Geometry check sheet. Reference: the model listing, model coordinates, mm. A direction names the side the tool comes from. Round coordinates to 2 decimals unless told otherwise and drop trailing zeros. Write each loop counter-clockwise with the first axis right and the second up, starting at its lowest first coordinate (ties: lowest second). Pieces come first, ordered by that corner, then holes.
from build123d import *

# Parameters (mm, degrees)
BOSS_EXTRUDE1_DEPTH = 18


with BuildPart() as part:
    # Sketch1 → Boss-Extrude1 (new body)
    with BuildSketch(Plane(origin=(0, 0, 0), x_dir=(1, 0, 0), z_dir=(0, 1, 0))):
        with BuildLine():
            Line((66.981499187, 102), (316.981499187, 102))
            Line((316.981499187, 102), (316.981499187, -38))
            Line((316.981499187, -38), (-83.018500813, -38))
            Line((-83.018500813, -38), (-83.018500813, 0))
            Line((-83.018500813, 0), (41.981499187, 0))
            ThreePointArc((41.981499187, 0), (59.659168717, 7.32233047), (66.981499187, 25))
            Line((66.981499187, 25), (66.981499187, 102))
        make_face()
    extrude(amount=BOSS_EXTRUDE1_DEPTH)


solid = part.part
1. Depth check by flat-ended pin: pin 1 Ø9 at (y, z) = (9.5, -77) entering from -X; pin 2 Ø10 at (x, z) = (160, 10) entering from -Y; pin 3 Ø8 at (x, z) = (-18.5, -7.5) entering from -Y. Enter the tip coordinate at first touch or a pass-through.
2. Section check B-B (x = 33). Record the cut outline in (y, z), plus the area to 3 significant figures.
3. Section check A-A (y = 11). Record the cut outline in (x, z), plus the area to 3 significant figures.
4. Section check C-C (z = -55.5). Record the cut outline in (x, y).
5. Access from +Z, -Z, +X, -X, +Y, -Y to the whole of each face (thin tool, end or side, straight path). Record for faces 1 (the face through (316.981, 9, -33)), 2 (the face through (66.981, 9, -63)).
6. Scan lines: line 1 along Z through (x, y) = (-47, 8); line 2 along X through (y, z) = (16.25, -27); line 3 along X through (y, z) = (7.25, -5). Record each from-to range of solid material in increasing order.
Results below:
1. pin 1: stops at x = 66.98
1. pin 2: stops at y = 0
1. pin 3: passes through
2. outline: (0, 0) - (18, 0) - (18, 38) - (0, 38) - close
2. area: 684 mm2
3. outline: (-83.02, 0) - (41.98, 0) arc R25 cw to (66.98, -25) - (66.98, -102) - (316.98, -102) - (316.98, 38) - (-83.02, 38) - close
3. area: 40,800 mm2
4. outline: (66.98, 0) - (316.98, 0) - (316.98, 18) - (66.98, 18) - close
5. face 1: +Z, -Z, +X, +Y, -Y
5. face 2: -Z, -X, +Y, -Y
6. line 1: z = 0 to 38
6. line 2: x = 66.98 to 316.98
6. line 3: x = 56.98 to 316.98
